from build123d import *

# Parameters (mm, degrees)
CROQUIS1_R                                           = 21.825
SALIENTE_EXTRUIR1_DEPTH                              = 4.5
CROQUIS2_R                                           = 2.5
SALIENTE_EXTRUIR2_DEPTH                              = 12
TALADRO_DE_MARGEN_PARA_M121_D                        = 13.5
SALIENTE_EXTRUIR3_DEPTH                              = 12
CROQUIS8_R                                           = 1.7
CORTAR_EXTRUIR1_DEPTH                                = 16.5
MATRIZC1_COUNT                                       = 3
TALADRO_DE_MARGEN_PARA_M21_D                         = 2.4
SALIENTE_EXTRUIR5_DEPTH                              = 4.5
MATRIZC2_COUNT                                       = 3
CROQUIS12_R                                          = 2.875
CORTAR_EXTRUIR2_DEPTH                                = 2.2
CROQUIS13_R                                          = 3
CORTAR_EXTRUIR3_DEPTH                                = 16.5
REFRENTADO_PARA_TORNILLO_CON_CABEZA_PLAN_D           = 3.4
REFRENTADO_PARA_TORNILLO_CON_CABEZA_PLAN_CBORE_D     = 6.5
REFRENTADO_PARA_TORNILLO_CON_CABEZA_PLAN_CBORE_DEPTH = 10


with BuildPart() as part:
    # Croquis1 → Saliente-Extruir1 (new body)
    with BuildSketch(Plane(origin=(0, 0, 0), x_dir=(1, 0, 0), z_dir=(0, 1, 0))):
        Circle(CROQUIS1_R)
    extrude(amount=SALIENTE_EXTRUIR1_DEPTH)

    # Croquis2 → Saliente-Extruir2 (add)
    with BuildSketch(Plane(origin=(0, 4.5, 0), x_dir=(1, 0, 0), z_dir=(0, 1, 0))):
        with Locations((0, 15)):
            Circle(CROQUIS2_R)
        with Locations((12.990381057, -7.5)):
            Circle(CROQUIS2_R)
        with Locations((-12.990381057, -7.5)):
            Circle(CROQUIS2_R)
    extrude(amount=SALIENTE_EXTRUIR2_DEPTH)

    # Taladro de margen para M121 (through all)
    with Locations(Plane(origin=(0, 4.5, 0), x_dir=(1, 0, 0), z_dir=(0, 1, 0))):
        with Locations((0, 0)):
            Hole(TALADRO_DE_MARGEN_PARA_M121_D / 2)

    # Croquis5 → Saliente-Extruir3 (add)
    with BuildSketch(Plane(origin=(0, 4.5, 0), x_dir=(1, 0, 0), z_dir=(0, 1, 0))):
        with BuildLine():
            ThreePointArc((-7.642674188, 4.4125), (-11.035446071, 10.994501306), (-11.800237164, 18.359875487))
            ThreePointArc((-11.800237164, 18.359875487), (-18.901004438, 10.9125), (-21.800237164, 1.039367411))
            ThreePointArc((-21.800237164, 1.039367411), (-15.039240468, 4.059725986), (-7.642674188, 4.4125))
        make_face()
    saliente_extruir3 = extrude(amount=SALIENTE_EXTRUIR3_DEPTH)

    # Croquis8 → Cortar-Extruir1 (cut)
    with BuildSketch(Plane(origin=(0, 16.5, 0), x_dir=(1, 0, 0), z_dir=(0, 1, 0))):
        with Locations((-14.722431864, 8.5)):
            Circle(CROQUIS8_R)
    cortar_extruir1 = extrude(amount=-CORTAR_EXTRUIR1_DEPTH, mode=Mode.SUBTRACT)

    # MatrizC1: Saliente-Extruir3, Cortar-Extruir1 ×3 about axis
    matrizc1_axis = Axis((0, 0, 0), (0, 1, 0))
    for i in range(1, MATRIZC1_COUNT):
        add(saliente_extruir3.rotate(matrizc1_axis, i * 360 / MATRIZC1_COUNT))
        add(cortar_extruir1.rotate(matrizc1_axis, i * 360 / MATRIZC1_COUNT), mode=Mode.SUBTRACT)

    # Taladro de margen para M21 (through all)
    with Locations(Plane(origin=(0, 16.5, 0), x_dir=(1, 0, 0), z_dir=(0, 1, 0))):
        with Locations((12.990381057, -7.5), (-12.990381057, -7.5), (0, 15)):
            Hole(TALADRO_DE_MARGEN_PARA_M21_D / 2)

    # Croquis11 → Saliente-Extruir5 (add)
    with BuildSketch(Plane.XZ):
        with BuildLine():
            ThreePointArc((-10, 19.399242898), (-18.901004438, 10.9125), (-21.800237164, -1.039367411))
            ThreePointArc((-21.800237164, -1.039367411), (-23.615858472, 13.634622246), (-10, 19.399242898))
        make_face()
    saliente_extruir5 = extrude(amount=-SALIENTE_EXTRUIR5_DEPTH)

    # MatrizC2: Saliente-Extruir5 ×3 about axis
    matrizc2_axis = Axis((0, 0, 0), (0, 1, 0))
    for i in range(1, MATRIZC2_COUNT):
        add(saliente_extruir5.rotate(matrizc2_axis, i * 360 / MATRIZC2_COUNT))

    # Croquis12 → Cortar-Extruir2 (cut)
    with BuildSketch(Plane.XZ):
        with Locations((-12.990381057, 7.5)):
            Circle(CROQUIS12_R)
        with Locations((12.990381057, 7.5)):
            Circle(CROQUIS12_R)
        with Locations((0, -15)):
            Circle(CROQUIS12_R)
    extrude(amount=-CORTAR_EXTRUIR2_DEPTH, mode=Mode.SUBTRACT)

    # Croquis13 → Cortar-Extruir3 (cut)
    with BuildSketch(Plane.XZ):
        with Locations((15.5, -15.5)):
            Circle(CROQUIS13_R)
        with Locations((-15.5, -15.5)):
            Circle(CROQUIS13_R)
        with Locations((-15.5, 15.5)):
            Circle(CROQUIS13_R)
        with Locations((15.5, 15.5)):
            Circle(CROQUIS13_R)
    extrude(amount=-CORTAR_EXTRUIR3_DEPTH, mode=Mode.SUBTRACT)

    # Refrentado para tornillo con cabeza plana de M31 (through all)
    with Locations(Plane(origin=(0, 16.5, 0), x_dir=(1, 0, 0), z_dir=(0, 1, 0))):
        with Locations((-14.722431864, 8.5), (0, -17), (14.722431864, 8.5)):
            CounterBoreHole(REFRENTADO_PARA_TORNILLO_CON_CABEZA_PLAN_D / 2, REFRENTADO_PARA_TORNILLO_CON_CABEZA_PLAN_CBORE_D / 2, REFRENTADO_PARA_TORNILLO_CON_CABEZA_PLAN_CBORE_DEPTH)


solid = part.part
Could you check a few things on this model? Use its own coordinates, in mm. A direction names the side the tool comes from. Coordinates: 2 decimals unless noted, no trailing zeros. Order: outer loops, then holes, each group sorted by start corner. A loop starts at its lowest first (then second) coordinate and runs counter-clockwise, first axis right, second up.
Q1. Please list where these lines run through material, in increasing order: L1, parallel to X at y = 1.5, z = -7.5; L2, parallel to Z at x = 15.5, y = 3.6; L3, parallel to X at y = 13.5, z = -15.
Q2. Suppose I cut it at B-B on x = -6. Please give me the cut outline in (y, z), and give its area (3 significant figures).
Q3. Suppose I cut it at C-C on z = 7.5. Please give me the cut outline in (x, y).
Q4. Suppose I cut it at D-D on z = 0. Please give me the cut outline in (x, y), and give its area (3 significant figures).
Q5. Will these pins go through, and if not, where does the flat tip stop? pin 1 (8 mm diameter, centred on x = 6.5, y = 3.5, fed in from +Z); pin 2 (1.5 mm diameter, centred on x = -11.5, z = 7.5, fed in from -Y); pin 3 (3 mm diameter, centred on y = 8, z = -14, fed in from +X); pin 4 (11 mm diameter, centred on x = 0, z = 0, fed in from -Y).
Q6. Which directions (+Z, -Z, +X, -X, +Y, -Y) give clear straight access to the entire face, cutting with the end or side of a thin tool? Please do faces 1 (the cylindrical face through (-0.54, 10.42, -12.56)), 2 (the flat face through (-1, 16.5, -14)), 3 (the cylindrical face through (10.71, 1.08, 5.75)).
Q7. Thinking about a two-plate mould opening in Z: for faces 4 (the cylindrical face through (-0.623, 1.085, -17.807)), 5 (the flat face through (-15, 16.5, -5)), 6 (the cylindrical face through (-23.725, 2.218, 13.441)), which applies, released by +Z, released by -Z, zero draft, split by the parting line, or undercut?
Q8. Suppose I cut it at A-A on y = 15. Give the number of separate pieces and of enclosed holes in the cut face, and give its area (3 significant figures).
Answer:
1. L1: x = -20.5 to -16.1, -13.35 to 13.35, 16.1 to 20.5
1. L2: z = -12.5 to -10.01, -6.99 to 12.5, 18.5 to 19.51
1. L3: x = -12.54 to -11.8, -2.5 to -1.2, 1.2 to 2.5, 11.8 to 12.54
2. outline: (0, -25.7) - (4.5, -25.7) - (4.5, -3.09) - (0, -3.09) - close; (0, 3.09) - (4.5, 3.09) - (4.5, 16.9) - (16.5, 16.9) - (16.5, 20.98) - (0, 20.98) - close
2. area: 231 mm2
3. outline: (-25.26, 0) - (-15.87, 0) - (-15.87, 2.2) - (-14.19, 2.2) - (-14.19, 16.5) - (-15.49, 16.5) - (-15.49, 4.5) - (-25.26, 4.5) - close; (-11.79, 2.2) - (-10.12, 2.2) - (-10.12, 0) - (10.12, 0) - (10.12, 2.2) - (11.79, 2.2) - (11.79, 16.5) - (10.49, 16.5) - (10.49, 4.5) - (-10.49, 4.5) - (-10.49, 16.5) - (-11.79, 16.5) - close; (14.19, 2.2) - (15.87, 2.2) - (15.87, 0) - (25.26, 0) - (25.26, 4.5) - (15.49, 4.5) - (15.49, 16.5) - (14.19, 16.5) - close
4. outline: (-22.7, 0) - (-6.75, 0) - (-6.75, 4.5) - (-22.7, 4.5) - close; (6.75, 0) - (22.7, 0) - (22.7, 4.5) - (6.75, 4.5) - close
4. area: 144 mm2
5. pin 1: stops at z = 21.68
5. pin 2: stops at y = 2.2
5. pin 3: stops at x = 17.89
5. pin 4: passes through
6. face 1: +Y
6. face 2: +Z, -Z, +X, -X, +Y
6. face 3: -Y
7. face 4: undercut
7. face 5: zero draft
7. face 6: split by the parting line
8. separate pieces: 6
8. enclosed holes: 6
8. area: 254 mm2
